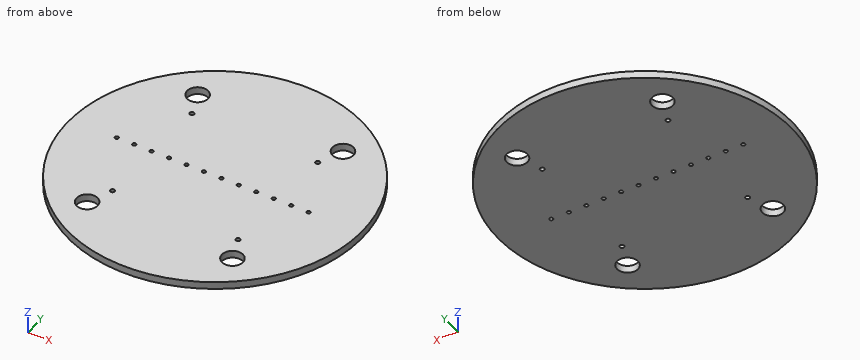
from build123d import *

# Parameters (mm, degrees)
F0_R     = 127
F0_R_2   = 9.0805
F0_R_3   = 1.905
F0_R_4   = 1.6002
F1_DEPTH = 6.35


with BuildPart() as f1:
    # F0 (on Top) → F1 (new body)
    with BuildSketch(Plane.XY):
        Circle(F0_R)
        with Locations((-63.5, -76.2)):
            Circle(F0_R_2, mode=Mode.SUBTRACT)
        with Locations((-54.9275, -54.9275)):
            Circle(F0_R_3, mode=Mode.SUBTRACT)
        with Locations((63.5, -76.2)):
            Circle(F0_R_2, mode=Mode.SUBTRACT)
        with Locations((54.9275, -54.9275)):
            Circle(F0_R_3, mode=Mode.SUBTRACT)
        with Locations((-86.36, 0.762)):
            Circle(F0_R_4, mode=Mode.SUBTRACT)
        with Locations((-71.12, 0.762)):
            Circle(F0_R_4, mode=Mode.SUBTRACT)
        with Locations((-55.88, 0.762)):
            Circle(F0_R_4, mode=Mode.SUBTRACT)
        with Locations((-40.64, 0.762)):
            Circle(F0_R_4, mode=Mode.SUBTRACT)
        with Locations((-25.4, 0.762)):
            Circle(F0_R_4, mode=Mode.SUBTRACT)
        with Locations((-10.16, 0.762)):
            Circle(F0_R_4, mode=Mode.SUBTRACT)
        with Locations((-54.9275, 54.9275)):
            Circle(F0_R_3, mode=Mode.SUBTRACT)
        with Locations((-63.5, 76.2)):
            Circle(F0_R_2, mode=Mode.SUBTRACT)
        with Locations((5.08, 0.762)):
            Circle(F0_R_4, mode=Mode.SUBTRACT)
        with Locations((20.32, 0.762)):
            Circle(F0_R_4, mode=Mode.SUBTRACT)
        with Locations((35.56, 0.762)):
            Circle(F0_R_4, mode=Mode.SUBTRACT)
        with Locations((50.8, 0.762)):
            Circle(F0_R_4, mode=Mode.SUBTRACT)
        with Locations((54.9275, 54.9275)):
            Circle(F0_R_3, mode=Mode.SUBTRACT)
        with Locations((66.04, 0.762)):
            Circle(F0_R_4, mode=Mode.SUBTRACT)
        with Locations((81.28, 0.762)):
            Circle(F0_R_4, mode=Mode.SUBTRACT)
        with Locations((63.5, 76.2)):
            Circle(F0_R_2, mode=Mode.SUBTRACT)
    extrude(amount=F1_DEPTH)


solid = f1.part
Input: part model. Units: mm. Frame: model coordinates. Give positions to 0.01 mm unless a question says otherwise; leave off trailing zeros. Write each loop counter-clockwise with the first axis right and the second up, starting at its lowest first coordinate (ties: lowest second). Pieces come first, ordered by that corner, then holes.
Q1. Section A-A, the plane z = 2. State how many separate pieces and enclosed holes the cut face has, plus the area to 3 significant figures.
Q2. Material intervals for probe 1 along X at (y, z) = (70, 2.5); probe 2 along Y at (x, z) = (2, 3.75); probe 3 along Y at (x, z) = (-53.5, 5), sorted ascending.
Q3. Section C-C, the plane y = -26. Output: boundary loops of the cut face in (x, z), plus the area to 3 significant figures.
Q4. Section B-B, the plane y = -63. Output: boundary loops of the cut face in (x, z).
Q5. First-contact query: P1, Ø1.5, axis at x = -46, z = 4, coming from the -Y side; P2, Ø2, axis at x = 73.5, z = 5.5, coming from the +Y side; P3, Ø2, axis at x = -54, z = 5, coming from the +Y side. Flat tips, straight axial feed; report the tip coordinate or a pass-through.
Filled in:
1. separate pieces: 1
1. enclosed holes: 20
1. area: 49,500 mm2
2. probe 1: x = -105.97 to -70.13, -56.87 to 56.87, 70.13 to 105.97
2. probe 2: y = -126.98 to 126.98
2. probe 3: y = -115.18 to -56.19, -53.67 to 53.67, 56.19 to 115.18
3. outline: (-124.31, 0) - (124.31, 0) - (124.31, 6.35) - (-124.31, 6.35) - close
3. area: 1,580 mm2
4. outline: (-110.27, 0) - (110.27, 0) - (110.27, 6.35) - (-110.27, 6.35) - close
5. P1: stops at y = -118.67
5. P2: stops at y = 104.27
5. P3: stops at y = 115.41
